```python
from build123d import *

# Parameters (mm, degrees)
BOSS_EXTRUDE1_DEPTH           = 40.64
F_8_0_199_DIAMETER_HOLE1_D    = 5.0546
SKETCH7_R                     = 6.35
CUT_EXTRUDE1_DEPTH            = 40.64
TAP_DRILL_FOR_M3_5X0_6_TAP1_D = 2.9


with BuildPart() as part:
    # Sketch4 → Boss-Extrude1 (new body)
    with BuildSketch(Plane.XY):
        Polygon((14.300746269, 21.994029851), (20.650746269, 21.994029851), (20.650746269, -28.805970149), (9.223880597, -28.805970149), (-30.149253731, -28.805970149), (-30.149253731, -22.455970149), (14.300746269, -22.455970149), align=None)
    extrude(amount=BOSS_EXTRUDE1_DEPTH)

    # #8 (0.199) Diameter Hole1 (through all)
    with Locations(Plane(origin=(20.650746269, 0, 0), x_dir=(0, 0, -1), z_dir=(1, 0, 0))):
        with Locations((-20.32, -7.215970149)):
            Hole(F_8_0_199_DIAMETER_HOLE1_D / 2)

    # Sketch7 → Cut-Extrude1 (cut)
    with BuildSketch(Plane(origin=(0, -22.455970149, 0), x_dir=(1, 0, 0), z_dir=(0, 1, 0))):
        with Locations(Location((-19.033752527, -20.32, 0), (0, 0, 180))):
            Circle(SKETCH7_R)
    extrude(amount=-CUT_EXTRUDE1_DEPTH, mode=Mode.SUBTRACT)

    # Tap Drill for M3.5x0.6 Tap1 (through all)
    with Locations(Plane(origin=(0, -22.455970149, 0), x_dir=(1, 0, 0), z_dir=(0, 1, 0))):
        with Locations((-25.715782321, -11.007082392), (-25.837741258, -29.421678533), (-9.951212668, -38.73459614), (-9.707294794, -1.90540386), (6.179233795, -11.218321467), (6.057274858, -29.632917608)):
            Hole(TAP_DRILL_FOR_M3_5X0_6_TAP1_D / 2)


solid = part.part
```
Can you work these out from the model? Positions are in its coordinate system, mm. A direction names the side the tool comes from. Coordinates: 2 decimals unless noted, no trailing zeros. Order: outer loops, then holes, each group sorted by start corner. A loop starts at its lowest first (then second) coordinate and runs counter-clockwise, first axis right, second up. Notation, with made-up numbers: (59, 15.5) - (76, 15.5) arc R23 ccw to (76, 43.5) - close; hole circle Ø9 at (36, 32.25). An arc over 180 degrees is marked (long way). Answer in a Markdown table with one row per item.
1. If I drill on line 1 along X through (y, z) = (-26.5, 11); line 2 along X through (y, z) = (11, 7.5); line 3 along Y through (x, z) = (3, 38.5), over which ranges is the centre line in solid material (lowest first)?
Reply:
| item | result |
|---|---|
| line 1 | x = -30.15 to -27.17, -24.27 to 4.75, 7.61 to 20.65 |
| line 2 | x = 14.3 to 20.65 |
| line 3 | y = -28.81 to -22.46 |
2. Suppose I cut it at A-A (z = 20.32). Please give me the cut outline in (x, y).
Reply:
| item | result |
|---|---|
| outline | (-30.15, -28.81) - (-25.38, -28.81) - (-25.38, -22.46) - (-30.15, -22.46) - close; (-12.68, -28.81) - (20.65, -28.81) - (20.65, -9.74) - (14.3, -9.74) - (14.3, -22.46) - (-12.68, -22.46) - close; (14.3, -4.69) - (20.65, -4.69) - (20.65, 21.99) - (14.3, 21.99) - close |
3. If we mould it in two halves opening along X, with no side actions, what happens to faces 3 (the cylindrical face through (17.431, -7.105, 17.795)), 4 (the flat face through (14.301, -1, 20)), 5 (the flat face through (20.651, -3, 20)), 6 (the cylindrical face through (5.28, -25.68, 28.41))? For each: pulls with the +X half, pulls with the -X half, needs draft (parallel to the pull), parting line crosses it, or undercut.
Reply:
| item | result |
|---|---|
| face 3 | needs draft |
| face 4 | pulls with the -X half |
| face 5 | pulls with the +X half |
| face 6 | undercut |
4. For pin 1 (3.5 mm diameter, centred on x = -25.72, z = 11.01, fed in from +Y); pin 2 (7.5 mm diameter, centred on x = -19.03, z = 20.32, fed in from -Y); pin 3 (12 mm diameter, centred on y = -0.5, z = 25.5, fed in from -X), each with a flat end and sliding along its axis, tell me the tip position at first contact or that it passes through.
Reply:
| item | result |
|---|---|
| pin 1 | stops at y = -22.46 |
| pin 2 | passes through |
| pin 3 | stops at x = 14.3 |
5. Suppose I cut it at D-D (z = 36). Please give me the cut outline in (x, y).
Reply:
| item | result |
|---|---|
| outline | (-30.15, -28.81) - (20.65, -28.81) - (20.65, 21.99) - (14.3, 21.99) - (14.3, -22.46) - (-30.15, -22.46) - close |
6. Suppose I cut it at B-B (x = -18). Please give me the cut outline in (y, z), and give its area (3 significant figures).
Reply:
| item | result |
|---|---|
| outline | (-28.81, 0) - (-22.46, 0) - (-22.46, 14.05) - (-28.81, 14.05) - close; (-28.81, 26.59) - (-22.46, 26.59) - (-22.46, 40.64) - (-28.81, 40.64) - close |
| area | 178 mm^2 |
7. Suppose I cut it at C-C (y = -18). Please give me the cut outline in (x, z).
Reply:
| item | result |
|---|---|
| outline | (14.3, 0) - (20.65, 0) - (20.65, 40.64) - (14.3, 40.64) - close |
8. For faces 1 (the flat face through (-8, -22.456, 20)), 2 (the cylindrical face through (4.796, -25.675, 10.783)), which set-ups out of +Z, -Z, +X, -X, +Y, -Y let a thin tool reach every point of the face, with its end or its side?
Reply:
| item | result |
|---|---|
| face 1 | +Z, -Z, -X, +Y |
| face 2 | +Y, -Y |
